The model under review builds one solid part; all positions refer to its coordinate system, in mm. A direction names the side the tool comes from. Coordinates: 2 decimals unless noted, no trailing zeros. Loops run counter-clockwise (first coordinate to the right, second up) from the corner with the lowest first, then second, coordinate; pieces in that order, holes last. Notation, with made-up numbers: M 7.25,82.5 L 20.25,82.5 A24 ccw 20.25,102.5 Z; hole C -20.5,61.5 d10. An arc over 180 degrees is marked long. Return JSON: item names as keys, results as strings.
```python
from build123d import *

# Parameters (mm, degrees)
F0_W     = 100
F0_H     = 100
F1_DEPTH = 50
F2_W     = 88.519738
F2_H     = 88.223688
F3_DEPTH = 45
F4_R     = 7.5
F5_DEPTH = 25


with BuildPart() as f1:
    # F0 (on Front) → F1 (new body)
    with BuildSketch(Plane.XZ):
        with Locations((3.404604, -5.325158)):
            Rectangle(F0_W, F0_H)
    extrude(amount=F1_DEPTH)

    # F2 (on face) → F3 (cut)
    with BuildSketch(Plane.XZ.offset(50)):
        with Locations((3.256578, -4.588816)):
            Rectangle(F2_W, F2_H)
    extrude(amount=-F3_DEPTH, mode=Mode.SUBTRACT)

    # F4 (on face) → F5 (cut)
    with BuildSketch(Plane.XZ.offset(5)):
        with Locations((-21.003291, 24.523028)):
            Circle(F4_R)
        with Locations((27.516447, 24.523028)):
            Circle(F4_R)
        with Locations((27.516447, -33.70066)):
            Circle(F4_R)
        with Locations((-21.003291, -33.70066)):
            Circle(F4_R)
    extrude(amount=-F5_DEPTH, mode=Mode.SUBTRACT)


solid = f1.part
```
1. Add section C-C on x = -34.5. Give the boundary of the cut face in (y, z).
Check values:
{"outline": "M -50,-55.33 L 0,-55.33 L 0,44.67 L -50,44.67 L -50,39.52 L -5,39.52 L -5,-48.7 L -50,-48.7 Z"}
2. Add section B-B on z = -36. Give the boundary of the cut face in (x, y).
Check values:
{"outline": "M -46.6,-50 L -41,-50 L -41,-5 L -28.14,-5 L -28.14,0 L -46.6,0 Z; M -13.86,-5 L 20.38,-5 L 20.38,0 L -13.86,0 Z; M 34.66,-5 L 47.52,-5 L 47.52,-50 L 53.4,-50 L 53.4,0 L 34.66,0 Z"}
3. Add section A-A on y = -32. Give the boundary of the cut face in (x, z).
Check values:
{"outline": "M -46.6,-55.33 L 53.4,-55.33 L 53.4,44.67 L -46.6,44.67 Z; hole M -41,-48.7 L 47.52,-48.7 L 47.52,39.52 L -41,39.52 Z"}
4. Machinability: for faces 1 (the face through (-46.595, -25, -6)), 2 (the face through (3, -28, 39.523)), which of the approach directions +Z, -Z, +X, -X, +Y, -Y give a long, thin tool a straight path to every point of the face, cutting with its end or side? Answer none if there is none.
Check values:
{"face 1": "+Z, -Z, -X, +Y, -Y", "face 2": "-Y"}
5. To check wall thickness, follow line 1 (Z direction, x = -6.5, y = -7.5); line 2 (X direction, y = -40.5, z = -14); line 3 (Y direction, x = -33, z = 32.5). State the ranges of each line that lie inside material, in increasing order.
Check values:
{"line 1": "-55.33 to -48.7, 39.52 to 44.67", "line 2": "-46.6 to -41, 47.52 to 53.4", "line 3": "-5 to 0"}
6. Insertion check: pin 1 Ø10 at (x, z) = (16, 17) entering from -Y; pin 2 Ø9 at (x, z) = (-21, 24.52) entering from -Y. Each pin has a flat end and moves straight along its axis. Give the tip position at first contact, or say it passes through.
Check values:
{"pin 1": "y = -5", "pin 2": "through"}
7. The part is to be moulded in two halves that separate along Z. For faces 3 (the face through (3, -25, -55.325)), 4 (the face through (3, -28, -48.701)), 5 (the face through (53.405, -25, -6)), 6 (the face through (3, -25, 44.675)), say which applies: released by +Z, released by -Z, zero draft, split by the parting line, or undercut.
Check values:
{"face 3": "released by -Z", "face 4": "undercut", "face 5": "zero draft", "face 6": "released by +Z"}
8. Add section D-D on z = -46.5. Give the boundary of the cut face in (x, y), plus the area to 3 significant figures.
Check values:
{"outline": "M -46.6,-50 L -41,-50 L -41,-5 L 47.52,-5 L 47.52,-50 L 53.4,-50 L 53.4,0 L -46.6,0 Z", "area": "1,020 mm²"}
